Check sheet for the modelled part. Datum: model origin and axes. Units: mm. Round coordinates to 2 decimals unless told otherwise and drop trailing zeros. Loops run counter-clockwise (first coordinate to the right, second up) from the corner with the lowest first, then second, coordinate; pieces in that order, holes last. Notation, with made-up numbers: (52.25, -24.5) -> (68.25, -24.5) arc R29 ccw to (68.25, 13.5) -> close; hole circle Ø1 at (-19.75, 79). An arc over 180 degrees is marked (long way). One line per question, with ' | ' between items.
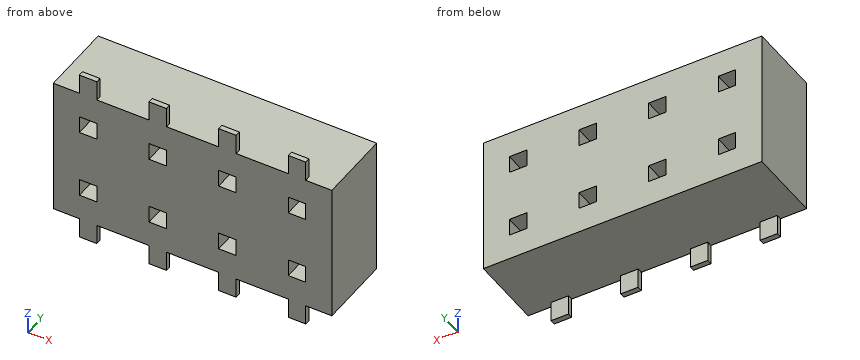
Autodesk Inventor part; units mm, degrees
ref_plane "YZ Plane" through (0, 0, 0) normal (1, 0, 0) x (0, 1, 0)
ref_plane "XZ Plane" through (0, 0, 0) normal (0, 1, 0) x (-1, 0, 0)
ref_plane "XY Plane" through (0, 0, 0) normal (0, 0, 1) x (1, 0, 0)
sketch "Sketch1" plane through (0, 0, 0) normal (0, 1, 0) x (-1, 0, 0)
  line L0 (-6.3636, 1.5475) -> (1.6364, 1.5475)
  line L1 (1.6364, 1.5475) -> (1.6364, -2.4525)
  line L2 (1.6364, -2.4525) -> (-6.3636, -2.4525)
  line L3 (-6.3636, -2.4525) -> (-6.3636, 1.5475)
  point P0 (0, 0)
  dimension "d0" = 4
  dimension "d1" = 8
extrude "Extrusion1" add sketch "Sketch1" along normal blind 2.13
sketch "Sketch3" plane through (0, 0, 0) normal (0, -1, 0) x (1, 0, 0)
  line L0 (6.3636, 1.5475) -> (-1.6364, 1.5475)
  line L1 (-1.6364, 1.5475) -> (-1.6364, -2.4525)
  line L2 (-0.8864, 2.1275) -> (-0.3864, 2.1275)
  line L3 (-0.3864, 2.1275) -> (-0.3864, -3.0325)
  line L4 (-0.3864, -3.0325) -> (-0.8864, -3.0325)
  line L5 (-0.8864, -3.0325) -> (-0.8864, 2.1275)
  point P0 (0, 0)
  dimension "d4" = 0.5
  dimension "d5" = 5.16
  dimension "d6" = 0.58
  dimension "d7" = 0.75
extrude "Extrusion2" add sketch "Sketch3" against normal blind 0.15
pattern_linear "Rectangular Pattern1" count 4 spacing 2 along (1, 0, 0) of "Extrusion2"
sketch "Sketch4" plane through (0, 2.13, 0) normal (0, 1, 0) x (1, 0, 0)
  line L0 (6.3636, 2.4525) -> (-1.6364, 2.4525)
  line L1 (-1.6364, 2.4525) -> (-1.6364, -1.5475)
  line L2 (-0.8864, 1.7025) -> (-0.3864, 1.7025)
  line L3 (-0.3864, 1.7025) -> (-0.3864, 1.2025)
  line L4 (-0.3864, 1.2025) -> (-0.8864, 1.2025)
  line L5 (-0.8864, 1.2025) -> (-0.8864, 1.7025)
  point P0 (0, 0)
  dimension "d13" = 0.5
  dimension "d14" = 0.5
  dimension "d15" = 0.75
  dimension "d16" = 0.75
extrude "Extrusion3" cut sketch "Sketch4" against normal through all
pattern_linear "Rectangular Pattern2" count 4 spacing 2 along (1, 0, 0) count 2 spacing 2 along (0, 0, 1) of "Extrusion3"
properties part number "2mm2Row8PosFemale"
(1) Sectioned sample at B-B, the plane x = 5.5. Record the cut outline in (y, z), and give its area (3 significant figures).
Answer:
outline: (0, -3.03) -> (0.15, -3.03) -> (0.15, -2.45) -> (2.13, -2.45) -> (2.13, -1.7) -> (0, -1.7) -> close; (0, -1.2) -> (2.13, -1.2) -> (2.13, 0.3) -> (0, 0.3) -> close; (0, 0.8) -> (2.13, 0.8) -> (2.13, 1.55) -> (0.15, 1.55) -> (0.15, 2.13) -> (0, 2.13) -> close | area: 6.56 mm2
(2) Scan lines: probe 1 along Z at (x, y) = (-0.5, 0.75); probe 2 along X at (y, z) = (1.85, -1.5); probe 3 along Z at (x, y) = (5.75, 0.55). Record each from-to range of solid material in increasing order.
Answer:
probe 1: z = -2.45 to -1.7, -1.2 to 0.3, 0.8 to 1.55 | probe 2: x = -1.64 to -0.89, -0.39 to 1.11, 1.61 to 3.11, 3.61 to 5.11, 5.61 to 6.36 | probe 3: z = -2.45 to 1.55
(3) Sectioned sample at C-C, the plane y = 0.8. Count the separate pieces of the cut face and the enclosed holes in it, and give its area (3 significant figures).
Answer:
separate pieces: 1 | enclosed holes: 8 | area: 30.0 mm2
(4) Sectioned sample at A-A, the plane z = 0.4. Record the cut outline in (x, y).
Answer:
outline: (-1.64, 0) -> (-0.89, 0) -> (-0.89, 2.13) -> (-1.64, 2.13) -> close; (-0.39, 0) -> (1.11, 0) -> (1.11, 2.13) -> (-0.39, 2.13) -> close; (1.61, 0) -> (3.11, 0) -> (3.11, 2.13) -> (1.61, 2.13) -> close; (3.61, 0) -> (5.11, 0) -> (5.11, 2.13) -> (3.61, 2.13) -> close; (5.61, 0) -> (6.36, 0) -> (6.36, 2.13) -> (5.61, 2.13) -> close
(5) Sectioned sample at D-D, the plane x = 0.5. Record the cut outline in (y, z).
Answer:
outline: (0, -2.45) -> (2.13, -2.45) -> (2.13, 1.55) -> (0, 1.55) -> close
